```python
from build123d import *

# Parameters (mm, degrees)
SKETCH_1_W               = 6.5
SKETCH_1_H               = 35
EXTRUDE_1_DEPTH          = 550
SKETCH_3_R               = 3
EXTRUDE_2_DEPTH          = 5
MIRROR_2_COPY_1_SKETCH_R = 3
MIRROR_2_COPY_1_DEPTH    = 5
CHAMFER_1_SIZE           = 1
CHAMFER_2_SIZE           = 1


with BuildPart() as part:
    # 草图1 → 凸台-拉伸1 (new body)
    with BuildSketch(Plane(origin=(0, 0, 0), x_dir=(0, 0, -1), z_dir=(1, 0, 0))):
        with Locations((3.25, -17.5)):
            Rectangle(SKETCH_1_W, SKETCH_1_H)
    extrude(amount=EXTRUDE_1_DEPTH)

    # 草图3 → 凸台-拉伸2 (add)
    with BuildSketch(Plane(origin=(450, 0, 0), x_dir=(0, 0, -1), z_dir=(1, 0, 0))):
        with BuildLine():
            Line((6.5, -21.25), (6.5, -13.75))
            Line((6.5, -13.75), (15.004809472, -13.75))
            ThreePointArc((15.004809472, -13.75), (29, -17.5), (15.004809472, -21.25))
            Line((15.004809472, -21.25), (6.5, -21.25))
        make_face()
        with Locations((21.5, -17.5)):
            Circle(SKETCH_3_R, mode=Mode.SUBTRACT)
    extrude_2 = extrude(amount=-EXTRUDE_2_DEPTH)

    # 镜向1: 凸台-拉伸2 across plane
    add(extrude_2.mirror(Plane.ZY.offset(-442.35)))

    # 镜向2: 凸台-拉伸2 across plane
    add(extrude_2.mirror(Plane(origin=(275, 0, 0), x_dir=(0, 0, 1), z_dir=(1, 0, 0))))

    # 镜向2 copy 1 sketch → 镜向2 copy 1 (add)
    with BuildSketch(Plane(origin=(115.3, 0, 0), x_dir=(0, 0, -1), z_dir=(1, 0, 0))):
        with BuildLine():
            Line((6.5, -21.25), (6.5, -13.75))
            Line((6.5, -13.75), (15.004809472, -13.75))
            ThreePointArc((15.004809472, -13.75), (29, -17.5), (15.004809472, -21.25))
            Line((15.004809472, -21.25), (6.5, -21.25))
        make_face()
        with Locations((21.5, -17.5)):
            Circle(MIRROR_2_COPY_1_SKETCH_R, mode=Mode.SUBTRACT)
    extrude(amount=-MIRROR_2_COPY_1_DEPTH)

    # 倒角1
    chamfer_1_edges = [part.edges().sort_by_distance(p)[0] for p in [
        (550, -17.5, -6.5),
        (550, 0, -3.25),
        (445, -17.5, -6.5),
        (447.5, -21.25, -6.5),
        (447.5, -13.75, -6.5),
        (445, -17.5, -18.5),
        (450, -17.5, -6.5),
        (450, -17.5, -18.5),
        (439.7, -17.5, -6.5),
        (434.7, -17.5, -18.5),
        (434.7, -17.5, -6.5),
        (437.2, -13.75, -6.5),
        (437.2, -21.25, -6.5),
        (439.7, -17.5, -18.5),
        (105, -17.5, -6.5),
        (100, -17.5, -6.5),
        (0, 0, -3.25),
        (102.5, -13.75, -6.5),
        (102.5, -21.25, -6.5),
        (0, -17.5, -6.5),
        (0, -35, -3.25),
        (110.3, -17.5, -6.5),
        (112.8, -21.25, -6.5),
        (112.8, -13.75, -6.5),
        (115.3, -17.5, -6.5),
        (275, 0, 0),
        (275, 0, -6.5),
        (275, -35, -6.5),
        (275, -35, 0),
        (550, -35, -3.25),
    ]]
    chamfer(chamfer_1_edges, length=CHAMFER_1_SIZE)

    # 倒角2
    chamfer_2_edges = [part.edges().sort_by_distance(p)[0] for p in [
        (100, -17.5, -18.5),
        (105, -17.5, -18.5),
        (110.3, -17.5, -18.5),
        (115.3, -17.5, -18.5),
    ]]
    chamfer(chamfer_2_edges, length=CHAMFER_2_SIZE)


solid = part.part
```
Geometry check sheet. Reference: the model listing, model coordinates, mm. A direction names the side the tool comes from. Give positions to 0.01 mm unless a question says otherwise; leave off trailing zeros. Order: outer loops, then holes, each group sorted by start corner. A loop starts at its lowest first (then second) coordinate and runs counter-clockwise, first axis right, second up.
1. Access from +Z, -Z, +X, -X, +Y, -Y to the whole of each face (thin tool, end or side, straight path). Record for faces 4 (the face through (437.165, -17.225, -28.995)), 5 (the face through (105, -17, -16)), 6 (the face through (100, -17, -16)).
2. Section check A-A, the plane x = 473.5. Enter the section's corners in (y, z).
3. Release check for a two-part mould opening along X. For faces 1 (the face through (434.7, -17, -16)), 2 (the face through (112.835, -17.225, -28.995)), 3 (the face through (450, -17, -16)) record: pulls with the +X half, pulls with the -X half, needs draft (parallel to the pull), parting line crosses it, or undercut.
4. Thickness scan on L1, parallel to X at y = -16, z = -8; L2, parallel to Y at x = 112.65, z = -21.5; L3, parallel to Z at x = 102, y = -17. Record the ranges inside material, lowest first.
5. Gauge pin test, flat ends, axial feed: pin 1 Ø12 at (y, z) = (-15, -21.5) entering from -X; pin 2 Ø1 at (x, y) = (318, -16) entering from -Z; pin 3 Ø16.5 at (y, z) = (-20, -18) entering from +X. Record the tip position at first contact, or that the pin passes through.
Values follow:
1. face 4: +X, -X
1. face 5: -Z, +Y, -Y
1. face 6: -Z, -X, +Y, -Y
2. outline: (-35, -5.5) - (-34, -6.5) - (-1, -6.5) - (0, -5.5) - (0, -1) - (-1, 0) - (-34, 0) - (-35, -1) - close
3. face 1: undercut
3. face 2: needs draft
3. face 3: pulls with the +X half
4. L1: x = 100 to 105, 110.3 to 115.3, 434.7 to 439.7, 445 to 450
4. L2: y = -25 to -20.5, -14.5 to -10
4. L3: z = -28.98 to -24.46, -18.54 to 0
5. pin 1: stops at x = 100
5. pin 2: stops at z = -6.5
5. pin 3: stops at x = 450
